Can you work these out from the model? Positions are in its coordinate system, mm. Face numbers are marked on the shaded views. A direction names the side the tool comes from. Give positions to 0.01 mm unless a question says otherwise; leave off trailing zeros. Order: outer loops, then holes, each group sorted by start corner. A loop starts at its lowest first (then second) coordinate and runs counter-clockwise, first axis right, second up.
Item 1: If we mould it in two halves opening along Z, with no side actions, what happens to the marked faces 1, 2 and 3? For each: +Z half, -Z half, draft (parallel to the pull), parting line (faces both ways), or undercut.
Item 2: I want a section at A-A, the plane x = 0. Write out the boundary of the cut face in (y, z).
Item 3: I want a section at C-C, the plane x = -3. Write out the boundary of the cut face in (y, z), then the cut area to 3 significant figures.
Item 4: I want a section at D-D, the plane z = 0. Write out the boundary of the cut face in (x, y), then the cut area to 3 significant figures.
Item 5: Which directions (+Z, -Z, +X, -X, +Y, -Y) give clear straight access to the entire face, cutting with the end or side of a thin tool? Please do the marked faces 4, 5 and 6.
Item 6: If I drill on line 1 along Z through (x, y) = (-4, 0.9); line 2 along Z through (x, y) = (0.25, 0.55); line 3 along X through (y, z) = (0.8, -4), over which ranges is the centre line in solid material (lowest first)?
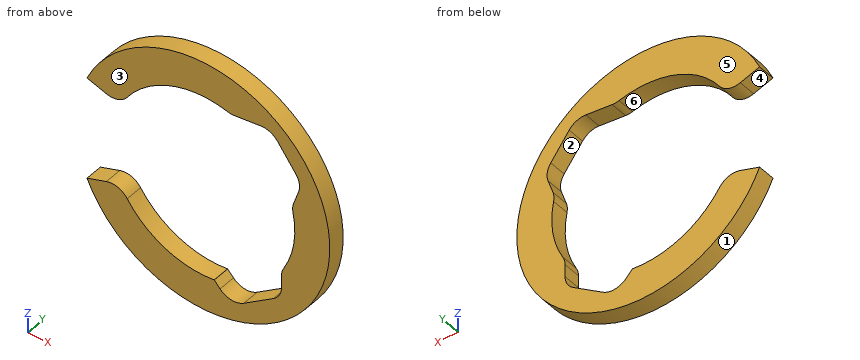
```python
from build123d import *

# Parameters (mm, degrees)
BOSS_EXTRUDE1_DEPTH = 0.94


with BuildPart() as part:
    # Sketch1 → Boss-Extrude1 (new body)
    with BuildSketch(Plane(origin=(0, 0, 0), x_dir=(1, 0, 0), z_dir=(0, 1, 0))):
        with BuildLine():
            Line((-5.253863679, -2.454338371), (-6.305884625, -2.801038932))
            ThreePointArc((-6.305884625, -2.801038932), (6.9, 0), (-6.305884625, 2.801038932))
            Line((-6.305884625, 2.801038932), (-5.253863679, 2.454338371))
            ThreePointArc((-5.253863679, 2.454338371), (-4.621952363, 2.45630843), (-4.117388267, 2.83674353))
            ThreePointArc((-4.117388267, 2.83674353), (-2.052207562, 4.559434627), (0.606687952, 4.963056491))
            Line((0.606687952, 4.963056491), (0.616921004, 4.961794884))
            Line((0.616921004, 4.961794884), (0.933263365, 5.299935719))
            ThreePointArc((0.933263365, 5.299935719), (1.550759285, 5.61038152), (2.222116774, 5.446195866))
            Line((2.222116774, 5.446195866), (3.835339689, 4.359739617))
            ThreePointArc((3.835339689, 4.359739617), (4.159519117, 4.000089674), (4.276739309, 3.53030269))
            Line((4.276739309, 3.53030269), (4.276739309, 2.855875044))
            ThreePointArc((4.276739309, 2.855875044), (4.307343479, 2.610372041), (4.397282758, 2.37989587))
            ThreePointArc((4.397282758, 2.37989587), (4.945409591, 0.736833755), (4.900068255, -0.994651244))
            ThreePointArc((4.900068255, -0.994651244), (4.882230643, -1.259101387), (4.934494135, -1.518948622))
            Line((4.934494135, -1.518948622), (5.202364417, -2.297438027))
            ThreePointArc((5.202364417, -2.297438027), (5.244325234, -2.78011945), (5.054466855, -3.22587259))
            Line((5.054466855, -3.22587259), (4.054517147, -4.548527481))
            ThreePointArc((4.054517147, -4.548527481), (3.653996144, -4.863205448), (3.150433841, -4.939784193))
            Line((3.150433841, -4.939784193), (1.714554284, -4.786144484))
            ThreePointArc((1.714554284, -4.786144484), (1.525879552, -4.783859514), (1.340134323, -4.817057193))
            ThreePointArc((1.340134323, -4.817057193), (-1.705489788, -4.700138783), (-4.117388267, -2.83674353))
            ThreePointArc((-4.117388267, -2.83674353), (-4.621952363, -2.45630843), (-5.253863679, -2.454338371))
        make_face()
    extrude(amount=BOSS_EXTRUDE1_DEPTH)


solid = part.part
```
Results list:
1. face 1: parting line
1. face 2: undercut
1. face 3: draft
2. outline: (0, -6.9) - (0.94, -6.9) - (0.94, -5) - (0, -5) - close; (0, 5) - (0.94, 5) - (0.94, 6.9) - (0, 6.9) - close
3. outline: (0, -6.21) - (0.94, -6.21) - (0.94, -4) - (0, -4) - close; (0, 4) - (0.94, 4) - (0.94, 6.21) - (0, 6.21) - close
3. area: 4.16 mm2
4. outline: (5, 0) - (6.9, 0) - (6.9, 0.94) - (5, 0.94) - close
4. area: 1.79 mm2
5. face 4: -X, +Y, -Y
5. face 5: +Z, -Z, +X, -X, +Y
5. face 6: +Y, -Y
6. line 1: z = -5.62 to -3, 3 to 5.62
6. line 2: z = -6.9 to -4.99, 4.99 to 6.9
6. line 3: x = -5.62 to -3, 4.16 to 5.62
